Input: part model. Units: mm. Frame: model coordinates. A direction names the side the tool comes from. Coordinates: 2 decimals unless noted, no trailing zeros. Loops run counter-clockwise (first coordinate to the right, second up) from the corner with the lowest first, then second, coordinate; pieces in that order, holes last. Notation, with made-up numbers: M 36,30.25 L 52,30.25 A25 ccw 52,61.25 Z; hole C 54.25,85.25 d2. An arc over 180 degrees is marked long. Use a Markdown table: item, result. Add a question column.
1. Set-up query: faces 5 (the flat face through (-1, 1, 20.926)), 6 (the flat face through (55.614, 72.248, 9.123)), 7 (the cylindrical face through (64.607, -15.456, -9.661)). Return all of +Z, -Z, +X, -X, +Y, -Y with unobstructed straight access to the full face (end or side cutting, diameter ignored); none if empty.
2. Line query: L1, parallel to Y at x = 0, z = 28.5; L2, parallel to Y at x = 0, z = 15; L3, parallel to Y at x = -26, z = -4. Output: solid intervals per line, ascending. Write a range as [from, to].
3. Draft query along X for faces 1 (the flat face through (-55.614, -72.248, 9.123)), 2 (the cylindrical face through (-5.243, 39.935, 28.653)), 3 (the cylindrical face through (87.898, 0.196, 9.123)), 4 (the cylindrical face through (-0.47, 146.27, 9.12)). Return one class per face: +X half, -X half, draft (parallel to the pull), parting line (faces both ways), or undercut.
4. Section B-B on x = 0. Output: boundary loops of the cut face in (y, z), then the cut area to 3 significant figures.
5. Section D-D on z = 14.5. Output: boundary loops of the cut face in (x, y).
6. Section C-C on y = 0. Output: boundary loops of the cut face in (x, z).
7. Section A-A on z = -12. Output: boundary loops of the cut face in (x, y).
8. Pin query (flat end, axial travel): pin 1 (1.5 mm diameter, centred on y = -34, z = -1, fed in from -X); pin 2 (2 mm diameter, centred on x = 67, z = -2, fed in from -Y); pin 3 (1.5 mm diameter, centred on x = -59.5, z = 30.5, fed in from -Y). Return the tip coordinate at first contact, or that it passes through.
```python
from build123d import *

# Parameters (mm, degrees)
BOSS_EXTRUDE1_DEPTH = 17.78
SKETCH2_R           = 13.426008181
CUT_EXTRUDE1_DEPTH  = 5.08
SCALE1_SCALE        = 1.5
SCALE2_SCALE        = 2
SKETCH3_R           = 25.4
CUT_EXTRUDE2_DEPTH  = 15.24


with BuildPart() as part:
    # Sketch1 → Boss-Extrude1 (new body)
    with BuildSketch(Plane.XY):
        with BuildLine():
            Line((-28.241863774, 4.513574723), (-9.102375691, 43.111542356))
            ThreePointArc((-9.102375691, 43.111542356), (0, 48.757967634), (9.102375691, 43.111542356))
            Line((9.102375691, 43.111542356), (28.241863774, 4.513574723))
            ThreePointArc((28.241863774, 4.513574723), (29.299488083, 0), (28.241863774, -4.513574723))
            Line((28.241863774, -4.513574723), (9.102375691, -43.111542356))
            ThreePointArc((9.102375691, -43.111542356), (0, -48.757967634), (-9.102375691, -43.111542356))
            Line((-9.102375691, -43.111542356), (-28.241863774, -4.513574723))
            ThreePointArc((-28.241863774, -4.513574723), (-29.299488083, 0), (-28.241863774, 4.513574723))
        make_face()
    extrude(amount=BOSS_EXTRUDE1_DEPTH)

    # Sketch2 → Cut-Extrude1 (cut)
    with BuildSketch(Plane.XY.offset(17.78)):
        Circle(SKETCH2_R)
    extrude(amount=-CUT_EXTRUDE1_DEPTH, mode=Mode.SUBTRACT)


with BuildPart() as part_1:
    # Scale1: scaled about (0, 0, 8.587002836)
    add(part.part.scale(SCALE1_SCALE).moved(Location((0, 0, -4.293501418))))


with BuildPart() as part_2:
    # Scale2: scaled about (0, 0, 8.587002836)
    add(part_1.part.scale(SCALE2_SCALE).moved(Location((0, 0, -8.587002836))))

    # Sketch3 → Cut-Extrude2 (cut)
    with BuildSketch(Plane(origin=(0, 0, -17.174005673), x_dir=(-1, 0, 0), z_dir=(0, 0, -1))):
        with Locations((-44.45, 0)):
            Circle(SKETCH3_R)
        with Locations((44.45, 0)):
            Circle(SKETCH3_R)
    extrude(amount=-CUT_EXTRUDE2_DEPTH, mode=Mode.SUBTRACT)


solid = part_2.part
```
Answers below:
| question | item | result |
|---|---|---|
| 1 | face 5 | +Z |
| 1 | face 6 | +Z, -Z, +X, +Y |
| 1 | face 7 | -Z |
| 2 | L1 | y = [-146.27, -40.28], [40.28, 146.27] |
| 2 | L2 | y = [-146.27, 146.27] |
| 2 | L3 | y = [-131.7, -17.46], [17.46, 131.7] |
| 3 | face 1 | -X half |
| 3 | face 2 | undercut |
| 3 | face 3 | +X half |
| 3 | face 4 | parting line |
| 4 | outline | M -146.27,-17.17 L 146.27,-17.17 L 146.27,36.17 L 40.28,36.17 L 40.28,20.93 L -40.28,20.93 L -40.28,36.17 L -146.27,36.17 Z |
| 4 | area | 14,400 mm² |
| 5 | outline | M -84.73,-13.54 L -27.31,-129.33 A30.48 ccw 27.31,-129.33 L 84.73,-13.54 A30.48 ccw 84.73,13.54 L 27.31,129.33 A30.48 ccw -27.31,129.33 L -84.73,13.54 A30.48 ccw Z |
| 6 | outline | M -87.9,-17.17 L -69.85,-17.17 L -69.85,-1.93 L -19.05,-1.93 L -19.05,-17.17 L 19.05,-17.17 L 19.05,-1.93 L 69.85,-1.93 L 69.85,-17.17 L 87.9,-17.17 L 87.9,36.17 L 40.28,36.17 L 40.28,20.93 L -40.28,20.93 L -40.28,36.17 L -87.9,36.17 Z |
| 7 | outline | M -84.73,-13.54 L -27.31,-129.33 A30.48 ccw 27.31,-129.33 L 84.73,-13.54 A30.48 ccw 84.73,13.54 L 27.31,129.33 A30.48 ccw -27.31,129.33 L -84.73,13.54 A30.48 ccw Z; hole C -44.45,0 d50.8; hole C 44.45,0 d50.8 |
| 8 | pin 1 | stops at x = -74.95 |
| 8 | pin 2 | stops at y = -51.3 |
| 8 | pin 3 | stops at y = -65.92 |
